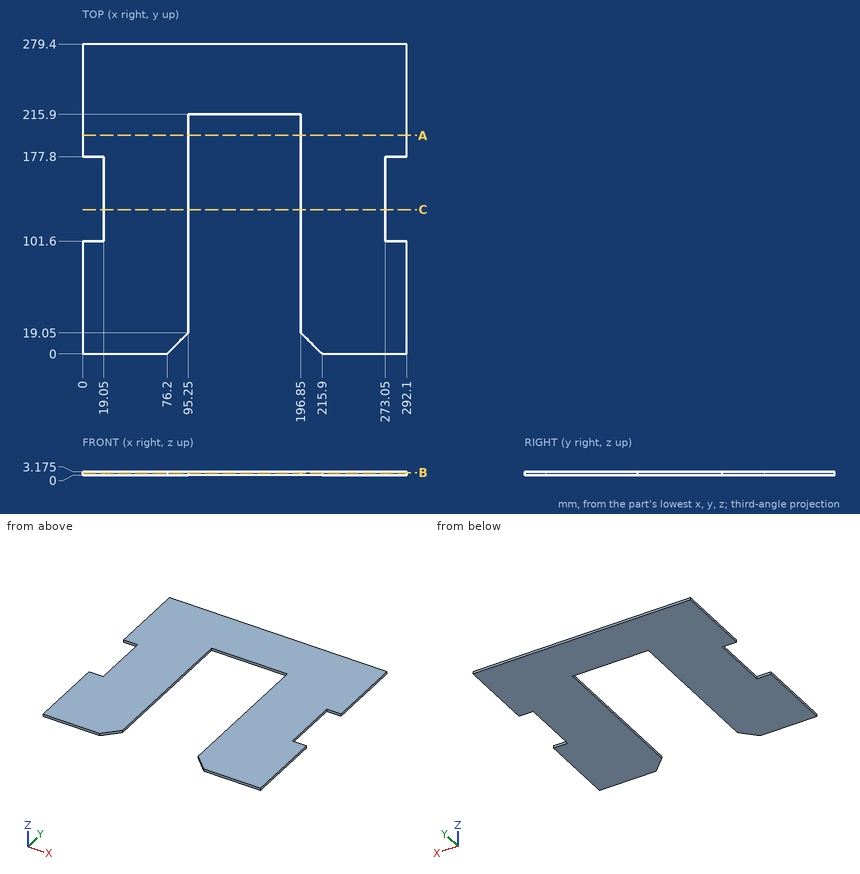
Study the drawing (mm; zero at the part's minimum x, y, z) and answer. Give positions to 0.01 mm unless a question says otherwise; leave off trailing zeros. Write each loop counter-clockwise with the first axis right and the second up, starting at its lowest first coordinate (ties: lowest second). Pieces come first, ordered by that corner, then holes. Notation, with made-up numbers: (14, 74) - (42, 74) arc R10 ccw to (42, 91) - close; hole circle Ø2 at (-17.5, -26.5). An arc over 180 degrees is marked (long way). Use CSV: the item, a comma, the result in double quotes. Start each with the question number.
(1) Find section A-A (y = 197). Give the vertices of the cut face in (x, z) (3 decimals), plus the area to 3 significant figures.
(2) Find section C-C (y = 130). Give the vertices of the cut face in (x, z) (3 decimals), plus the area to 3 significant figures.
(3) Find section B-B (z = 2.55). Give the vertices of the cut face in (x, y).
(4) Given P1, Ø1, axis at y = 142.5, z = 1.5, coming from the -X side; P2, Ø1.6, axis at y = 136, z = 1, coming from the +X side; P3, Ø1, axis at x = 135.5, z = 0.5, coming from the -Y side, each flat-ended and moving along its own axis, determine where each tip first touches the part or whether it passes through.
(5) Consider line 1 along X through (y, z) = (212.5, 2.8); line 2 along X through (y, z) = (120, 0.2); line 3 along Y through (x, z) = (126, 2.6). Determine where each line is inside the solid, lowest interval first.
Findings below:
1,outline,"(0, 0) - (95.25, 0) - (95.25, 3.175) - (0, 3.175) - close; (196.85, 0) - (292.1, 0) - (292.1, 3.175) - (196.85, 3.175) - close"
1,area,"605 mm2"
2,outline,"(19.05, 0) - (95.25, 0) - (95.25, 3.175) - (19.05, 3.175) - close; (196.85, 0) - (273.05, 0) - (273.05, 3.175) - (196.85, 3.175) - close"
2,area,"484 mm2"
3,outline,"(0, 0) - (76.2, 0) - (95.25, 19.05) - (95.25, 215.9) - (196.85, 215.9) - (196.85, 19.05) - (215.9, 0) - (292.1, 0) - (292.1, 101.6) - (273.05, 101.6) - (273.05, 177.8) - (292.1, 177.8) - (292.1, 279.4) - (0, 279.4) - (0, 177.8) - (19.05, 177.8) - (19.05, 101.6) - (0, 101.6) - close"
4,P1,"x = 19.05"
4,P2,"x = 273.05"
4,P3,"y = 215.9"
5,line 1,"0 to 95.25, 196.85 to 292.1"
5,line 2,"19.05 to 95.25, 196.85 to 273.05"
5,line 3,"215.9 to 279.4"
